Verification items for the finished model (mm, model axes). Face numbers are marked on the shaded views. A direction names the side the tool comes from. Coordinates: 2 decimals unless noted, no trailing zeros. Write each loop counter-clockwise with the first axis right and the second up, starting at its lowest first coordinate (ties: lowest second). Pieces come first, ordered by that corner, then holes. Notation, with made-up numbers: (-29, -21) -> (23, -21) arc R13 cw to (23, 4) -> close; hole circle Ø2 at (-33.75, 19). An arc over 180 degrees is marked (long way). Write item = value, one per line. Start each with the question number.
(1) Set-up check for the marked faces 1, 2 and 3: record each of +Z, -Z, +X, -X, +Y, -Y from which the full face is reachable in a straight line by a thin tool's end or side.
(2) Section check B-B (y = -3.25). Record the cut outline in (x, z), plus the area to 3 significant figures.
(3) Section check D-D (x = -8). Record the cut outline in (y, z).
(4) Material ranges on probe 1 along Y at (x, z) = (0, 3); probe 2 along X at (y, z) = (4.25, 6.75); probe 3 along Z at (x, y) = (8, 6.5), recorded low to high. Write a range as [from, to].
(5) Section check A-A (x = -3.5). Record the cut outline in (y, z).
(6) Section check C-C (z = 2.5). Record the cut outline in (x, y).
(7) Gauge pin test, flat ends, axial feed: pin 1 Ø2 at (x, z) = (-2, 5.5) entering from -Y; pin 2 Ø2 at (x, z) = (-3, 6) entering from +Y; pin 3 Ø1.5 at (y, z) = (2, 3.5) entering from -X. Record the tip position at first contact, or that the pin passes through.
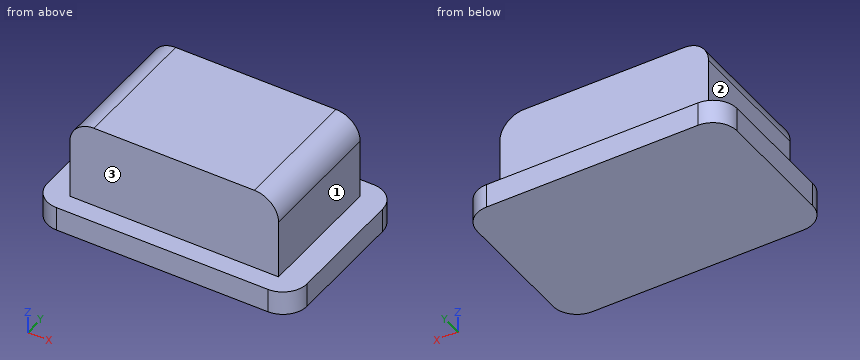
```python
from build123d import *

# Parameters (mm, degrees)
BOSS_EXTRUDE1_DEPTH = 2
SKETCH2_W           = 17.267499136
SKETCH2_H           = 10.808758156
BOSS_EXTRUDE2_DEPTH = 6.9
FILLET3_R           = 2


with BuildPart() as part:
    # Sketch1 → Boss-Extrude1 (new body)
    with BuildSketch(Plane.XY):
        with BuildLine():
            Line((-8.75, -7), (8.75, -7))
            ThreePointArc((8.75, -7), (10.164213562, -6.414213562), (10.75, -5))
            Line((10.75, -5), (10.75, 5))
            ThreePointArc((10.75, 5), (10.164213562, 6.414213562), (8.75, 7))
            Line((8.75, 7), (-8.75, 7))
            ThreePointArc((-8.75, 7), (-10.164213562, 6.414213562), (-10.75, 5))
            Line((-10.75, 5), (-10.75, -5))
            ThreePointArc((-10.75, -5), (-10.164213562, -6.414213562), (-8.75, -7))
        make_face()
    extrude(amount=BOSS_EXTRUDE1_DEPTH)

    # Sketch2 → Boss-Extrude2 (add)
    with BuildSketch(Plane.XY.offset(2)):
        Rectangle(SKETCH2_W, SKETCH2_H)
    extrude(amount=BOSS_EXTRUDE2_DEPTH)

    # Fillet3
    fillet3_edges = [part.edges().sort_by_distance(p)[0] for p in [
        (8.633749568, 0, 8.9),
        (-8.633749568, 0, 8.9),
    ]]
    fillet(fillet3_edges, radius=FILLET3_R)


solid = part.part
```
Response:
q1.face_1 = +Z, +X, +Y, -Y
q1.face_2 = +Z, -X, +Y, -Y
q1.face_3 = +Z, +X, -X, -Y
q2.outline = (-10.75, 0) -> (10.75, 0) -> (10.75, 2) -> (8.63, 2) -> (8.63, 6.9) arc R2 ccw to (6.63, 8.9) -> (-6.63, 8.9) arc R2 ccw to (-8.63, 6.9) -> (-8.63, 2) -> (-10.75, 2) -> close
q2.area = 160 mm2
q3.outline = (-7, 0) -> (7, 0) -> (7, 2) -> (5.4, 2) -> (5.4, 8.36) -> (-5.4, 8.36) -> (-5.4, 2) -> (-7, 2) -> close
q4.probe_1 = [-5.4, 5.4]
q4.probe_2 = [-8.63, 8.63]
q4.probe_3 = [0, 2]
q5.outline = (-7, 0) -> (7, 0) -> (7, 2) -> (5.4, 2) -> (5.4, 8.9) -> (-5.4, 8.9) -> (-5.4, 2) -> (-7, 2) -> close
q6.outline = (-8.63, -5.4) -> (8.63, -5.4) -> (8.63, 5.4) -> (-8.63, 5.4) -> close
q7.pin_1 = -5.4
q7.pin_2 = 5.4
q7.pin_3 = -8.63
